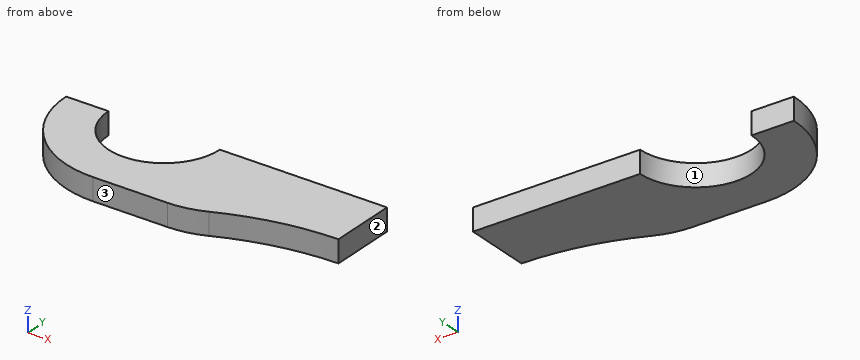
from build123d import *

# Parameters (mm, degrees)
SKETCH_R             = 12.5
PAD_DEPTH            = 5
SKETCH001_R          = 62.5
POCKET_DEPTH         = 5.001
POCKET_DEPTH_BACK    = -5.001
FILLET_R             = 20
POCKET001_DEPTH      = 5.001
POCKET001_DEPTH_BACK = -5.001
SKETCH003_W          = 72
SKETCH003_H          = 22
POCKET002_DEPTH      = 5.001


with BuildPart() as part:
    # Sketch → Pad (new body, symmetric)
    with BuildSketch(Plane.XY):
        with BuildLine():
            ThreePointArc((-50, 22), (-72, 0), (-50, -22))
            Line((-50, -22), (50, -22))
            ThreePointArc((50, -22), (72, 0), (50, 22))
            Line((50, 22), (-50, 22))
        make_face()
        with Locations((-50, 0)):
            Circle(SKETCH_R, mode=Mode.SUBTRACT)
        with Locations((50, 0)):
            Circle(SKETCH_R, mode=Mode.SUBTRACT)
    extrude(amount=PAD_DEPTH, both=True)

    # Sketch001 → Pocket (cut, two sides)
    with BuildSketch(Plane.XY) as pocket_sk:
        with Locations((0, -77.5)):
            Circle(SKETCH001_R)
        with Locations((0, 77.5)):
            Circle(SKETCH001_R)
    extrude(amount=-POCKET_DEPTH, mode=Mode.SUBTRACT)
    extrude(pocket_sk.sketch, amount=-POCKET_DEPTH_BACK, mode=Mode.SUBTRACT)

    # Fillet
    fillet_edges = [part.edges().sort_by_distance(p)[0] for p in [
        (-28.740216, -22, 0),
        (28.740216, -22, 0),
        (-28.740216, 22, 0),
        (28.740216, 22, 0),
    ]]
    fillet(fillet_edges, radius=FILLET_R)

    # Sketch002 → Pocket001 (cut, two sides)
    with BuildSketch(Plane.XY) as pocket001_sk:
        Polygon((72, -22), (72, 22), (-72, 22), (-72, 0), (0, 0), (0, -22), align=None)
    extrude(amount=-POCKET001_DEPTH, mode=Mode.SUBTRACT)
    extrude(pocket001_sk.sketch, amount=-POCKET001_DEPTH_BACK, mode=Mode.SUBTRACT)

    # Sketch003 → Pocket002 (cut, through all)
    with BuildSketch(Plane.XY):
        with Locations((-36, -11)):
            Rectangle(SKETCH003_W, SKETCH003_H)
    extrude(amount=-POCKET002_DEPTH, mode=Mode.SUBTRACT)


solid = part.part
Source: CAD feature listing. Evaluate the final solid. Frame: model axes, mm. Face numbers are marked on the shaded views. Coordinates: 2 decimals unless noted, no trailing zeros. Loops run counter-clockwise (first coordinate to the right, second up) from the corner with the lowest first, then second, coordinate; pieces in that order, holes last. Notation, with made-up numbers: (14.5, 29) - (46.5, 29) arc R31 cw to (46.5, 58) - close; hole circle Ø6 at (-16, -7). An arc over 180 degrees is marked (long way). One line per item, written item: value. Start each with the question number.
1. Ray query, L1, parallel to X at y = -3.5, z = 1.55; L2, parallel to Y at x = -33, z = 1.15; L3, parallel to X at y = -1.5, z = 4.05. Return the intervals inside material, ascending.
2. Section D-D (x = -64). Return the cut outline in (y, z), and give its area (3 significant figures).
3. Section B-B (z = 1.7). Return the cut outline in (x, y).
4. Contact query for flat-ended pins moving along their axis: P1, Ø1.5, axis at x = -49.5, z = 2.5, coming from the +Y side; P2, Ø2, axis at y = -13.5, z = 2.5, coming from the -X side. Output: stop coordinate, or through.
5. Mould query, pull axis X, two halves, no side actions, for the marked faces 1, 2 and 3. Classes: pulls with the +X half, pulls with the -X half, needs draft (parallel to the pull), parting line crosses it, or undercut.
6. Section A-A (y = -1.5). Return the cut outline in (x, z), and give its area (3 significant figures).
7. Section C-C (y = -11.25). Return the cut outline in (x, z), and give its area (3 significant figures).
Verdict:
1. L1: x = -71.72 to -62, -38 to 0
1. L2: y = -22 to 0
1. L3: x = -71.95 to -62.41, -37.59 to 0
2. outline: (-16.97, 0) - (0, 0) - (0, 5) - (-16.97, 5) - close
2. area: 84.9 mm2
3. outline: (-72, 0) arc R22 ccw to (-50, -22) - (-33.26, -22) arc R20 ccw to (-25.19, -20.3) arc R62.5 cw to (0, -15) - (0, 0) - (-37.5, 0) arc R12.5 cw to (-62.5, 0) - close
4. P1: stops at y = -12.44
4. P2: stops at x = -68.1
5. face 1: undercut
5. face 2: pulls with the +X half
5. face 3: needs draft
6. outline: (-71.95, 0) - (-62.41, 0) - (-62.41, 5) - (-71.95, 5) - close; (-37.59, 0) - (0, 0) - (0, 5) - (-37.59, 5) - close
6. area: 236 mm2
7. outline: (-68.91, 0) - (-55.45, 0) - (-55.45, 5) - (-68.91, 5) - close; (-44.55, 0) - (0, 0) - (0, 5) - (-44.55, 5) - close
7. area: 290 mm2
